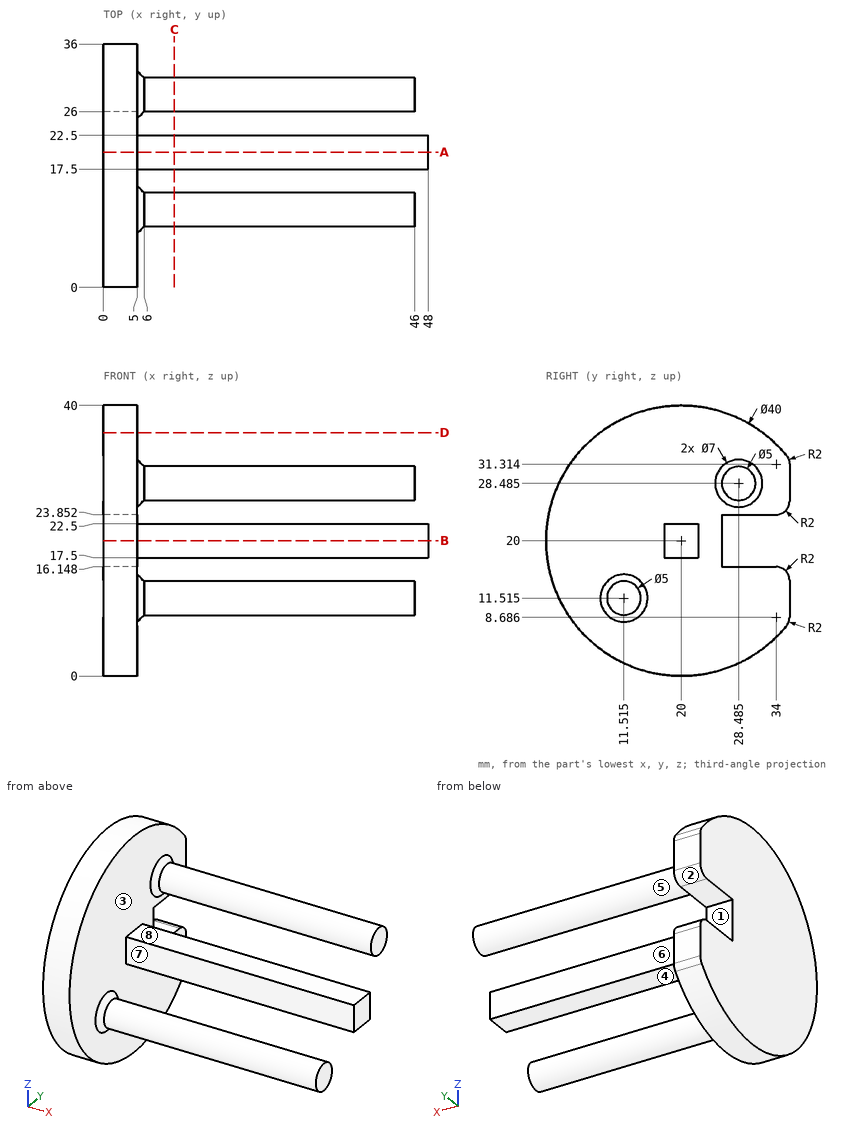
Print and shaded views of the part. All mm, measured from the part's lowest x, y and z. A direction names the side the tool comes from. Give positions to 0.01 mm unless a question says otherwise; leave off trailing zeros. Loops run counter-clockwise (first coordinate to the right, second up) from the corner with the lowest first, then second, coordinate; pieces in that order, holes last. Notation, with made-up numbers: (58, 74.25) -> (99, 74.25) arc R22 ccw to (99, 102.25) -> close; hole circle Ø3 at (77, 19). An arc over 180 degrees is marked (long way). One line per question, with ' | ' between items. Start each with the question number.
1) Cut at D-D (z = 36). Give the cut face in (x, y).
2) Probe L1, parallel to X at y = 22, z = 5; L2, parallel to Y at x = 31, z = 28.5 (1 decimal); L3, parallel to X at y = 28, z = 28.5. List the from-to ranges inside material, lowest first.
3) Two-plate mould, pull along Z, no slides. Class the marked faces 1, 2, 3 and 4: released by +Z, released by -Z, zero draft, split by the parting line, or undercut.
4) 3-axis set-ups, long thin cutter, end or side, ignore diameter. For the marked faces 5, 6, 7 and 8: which of +Z, -Z, +X, -X, +Y, -Y reach the whole face in a straight line?
5) Cut at A-A (y = 20). Give the cut face in (x, z).
6) Cut at B-B (z = 20). Give the cut face in (x, y).
7) Cut at C-C (x = 10.5). Give the cut face in (y, z) (1 decimal).
8) Pin check, flat tips, straight feed: pin 1 (2.5 mm diameter, centred on x = 29, y = 20, fed in from -Z); pin 2 (2.5 mm diameter, centred on x = 25, z = 19, fed in from -Y); pin 3 (5.5 mm diameter, centred on y = 12.5, z = 11.5, fed in from +X). Stop position of each tip, or through.
Return value:
1) outline: (0, 8) -> (5, 8) -> (5, 32) -> (0, 32) -> close
2) L1: 0 to 5 | L2: 26 to 31 | L3: 0 to 46
3) face 1: undercut | face 2: undercut | face 3: zero draft | face 4: released by -Z
4) face 5: +X | face 6: +Z, -Z, +X, +Y | face 7: +Z, -Z, +X, -Y | face 8: +Z, +X, +Y, -Y
5) outline: (0, 0) -> (5, 0) -> (5, 17.5) -> (48, 17.5) -> (48, 22.5) -> (5, 22.5) -> (5, 40) -> (0, 40) -> close
6) outline: (0, 0) -> (5, 0) -> (5, 17.5) -> (48, 17.5) -> (48, 22.5) -> (5, 22.5) -> (5, 26) -> (0, 26) -> close
7) outline: circle Ø5 at (11.5, 11.5); (17.5, 17.5) -> (22.5, 17.5) -> (22.5, 22.5) -> (17.5, 22.5) -> close; circle Ø5 at (28.5, 28.5)
8) pin 1: z = 17.5 | pin 2: y = 17.5 | pin 3: x = 46
